```python
from build123d import *

# Parameters (mm, degrees)
EXTRUDE_1_DEPTH     = 1.15
CUT_EXTRUDE_1_DEPTH = 1.23
EXTRUDE_2_DEPTH     = 1.35
CUT_EXTRUDE_START   = -10
CUT_EXTRUDE_2_DEPTH = 10
CUT_EXTRUDE_3_DEPTH = 1.35
FILLET_1_R          = 1.2


with BuildPart() as part:
    # 草图1 → 凸台-拉伸1 (new body)
    with BuildSketch(Plane.XY.offset(-0.646576548)):
        with BuildLine():
            Line((-91.3, 11.1), (-91.3, -11.1))
            Line((-91.3, -11.1), (-91.3, -14))
            ThreePointArc((-91.3, -14), (-91.252485776, -14.410844989), (-91.11245155, -14.8))
            Line((-91.11245155, -14.8), (-22.7, -14.8))
            Line((-22.7, -14.8), (-22.7, 14.8))
            Line((-22.7, 14.8), (-91.11245155, 14.8))
            ThreePointArc((-91.11245155, 14.8), (-91.252485776, 14.410844989), (-91.3, 14))
            Line((-91.3, 14), (-91.3, 11.1))
        make_face()
    extrude(amount=EXTRUDE_1_DEPTH)

    # 草图2 → 切除-拉伸1 (cut)
    with BuildSketch(Plane.XY.offset(0.503423452)):
        with BuildLine():
            Line((-91.4, 14), (-91.4, -14))
            ThreePointArc((-91.4, -14), (-91.342458697, -14.464053822), (-91.173320053, -14.9))
            Line((-91.173320053, -14.9), (-22.6, -14.9))
            Line((-22.6, -14.9), (-22.6, 14.9))
            Line((-22.6, 14.9), (-91.173320053, 14.9))
            ThreePointArc((-91.173320053, 14.9), (-91.342458697, 14.464053822), (-91.4, 14))
        make_face()
        with BuildLine():
            Line((-91.2, 14), (-91.2, -14))
            ThreePointArc((-91.2, -14), (-91.161870734, -14.358030253), (-91.049193338, -14.7))
            Line((-91.049193338, -14.7), (-22.8, -14.7))
            Line((-22.8, -14.7), (-22.8, 14.7))
            Line((-22.8, 14.7), (-91.049193338, 14.7))
            ThreePointArc((-91.049193338, 14.7), (-91.161870734, 14.358030253), (-91.2, 14))
        make_face(mode=Mode.SUBTRACT)
    extrude(amount=-CUT_EXTRUDE_1_DEPTH, mode=Mode.SUBTRACT)

    # 草图4 → 凸台-拉伸2 (add)
    with BuildSketch(Plane.XY.offset(0.503423452)):
        Polygon((-91.2, 13.700440852), (-23.8, 13.799558499), (-23.8, -13.799558499), (-91.2, -13.700440852), align=None)
    extrude(amount=EXTRUDE_2_DEPTH)

    # 草图5 → 切除-拉伸2 (cut)
    with BuildSketch(Plane(origin=(0, 0, -0.646576548), x_dir=(-1, 0, 0), z_dir=(0, 0, -1)).offset(CUT_EXTRUDE_START)):
        with BuildLine():
            Line((91.049193338, 14.7), (22.8, 14.7))
            Line((22.8, 14.7), (22.8, -14.7))
            Line((22.8, -14.7), (91.049193338, -14.7))
            ThreePointArc((91.049193338, -14.7), (91.161870734, -14.358030253), (91.2, -14))
            Line((91.2, -14), (91.2, 14))
            ThreePointArc((91.2, 14), (91.161870734, 14.358030253), (91.049193338, 14.7))
        make_face()
        with BuildLine():
            Line((90.914213562, 14.5), (23, 14.5))
            Line((23, 14.5), (23, -14.5))
            Line((23, -14.5), (90.914213562, -14.5))
            ThreePointArc((90.914213562, -14.5), (90.978397839, -14.253652968), (91, -14))
            Line((91, -14), (91, 14))
            ThreePointArc((91, 14), (90.978397839, 14.253652968), (90.914213562, 14.5))
        make_face(mode=Mode.SUBTRACT)
    extrude(amount=CUT_EXTRUDE_2_DEPTH, mode=Mode.SUBTRACT)

    # 草图6 → 切除-拉伸3 (cut)
    with BuildSketch(Plane.XY.offset(1.853423452)):
        Polygon((-24, 13.599264165), (-90.8, 13.501028871), (-91, 13.501028871), (-91, 13.70073497), (-23.8, 13.799558499), (-23.8, -13.799558499), (-91, -13.70073497), (-91, -13.501028871), (-90.8, -13.501028871), (-24, -13.599264165), align=None)
    extrude(amount=-CUT_EXTRUDE_3_DEPTH, mode=Mode.SUBTRACT)

    # 圆角1
    fillet_1_edges = [part.edges().sort_by_distance(p)[0] for p in [
        (-91, 0, 1.853423452),
    ]]
    fillet(fillet_1_edges, radius=FILLET_1_R)


solid = part.part
```
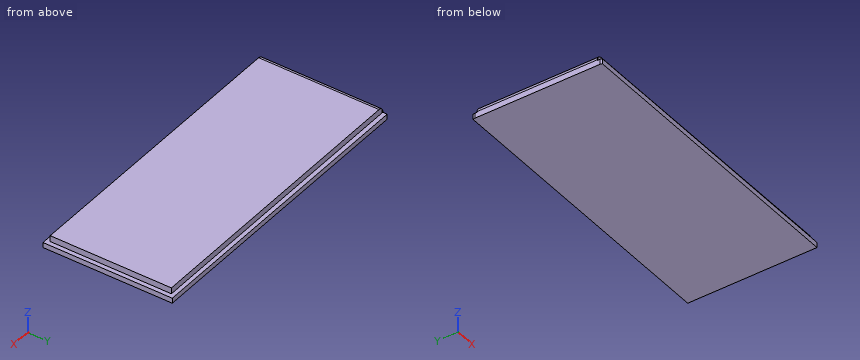
Check sheet for the modelled part. Datum: model origin and axes. Units: mm. Coordinates: 2 decimals unless noted, no trailing zeros. Loops run counter-clockwise (first coordinate to the right, second up) from the corner with the lowest first, then second, coordinate; pieces in that order, holes last.
1) Sectioned sample at B-B (x = -44.5). Record the boundary of the cut face in (y, z), and give its area (3 significant figures).
2) Material ranges on probe 1 along Y at (x, z) = (-83, 0.65); probe 2 along X at (y, z) = (10, 0.6); probe 3 along Y at (x, z) = (-34.5, 1.45), recorded low to high.
3) Sectioned sample at A-A (x = -28). Record the boundary of the cut face in (y, z), and give its area (3 significant figures).
Check sheet entries:
1. outline: (-14.5, -0.65) - (14.5, -0.65) - (14.5, 0.5) - (13.57, 0.5) - (13.57, 1.85) - (-13.57, 1.85) - (-13.57, 0.5) - (-14.5, 0.5) - close
1. area: 70.0 mm2
2. probe 1: y = -13.51 to 13.51
2. probe 2: x = -91 to -24
2. probe 3: y = -13.58 to 13.58
3. outline: (-14.5, -0.65) - (14.5, -0.65) - (14.5, 0.5) - (13.59, 0.5) - (13.59, 1.85) - (-13.59, 1.85) - (-13.59, 0.5) - (-14.5, 0.5) - close
3. area: 70.1 mm2
